from build123d import *

# Parameters (mm, degrees)
F1_DEPTH = 36
F3_DEPTH = 36
F4_R     = 14
F4_W     = 18
F4_H     = 16
F5_DEPTH = 44


with BuildPart() as f1:
    # F0 (on Front) → F1 (new body)
    with BuildSketch(Plane.XZ):
        Polygon((0, 44), (0, 0), (45, 0), (45, 13), (20, 27), (20, 44), align=None)
        Polygon((-45, 0), (0, 0), (0, 44), (-20, 44), (-20, 27), (-45, 13), align=None)
    extrude(amount=-F1_DEPTH)

    # F2 (on face) → F3 (cut)
    with BuildSketch(Plane.XZ):
        with BuildLine():
            Line((-20, 0), (20, 0))
            ThreePointArc((20, 0), (0, 20), (-20, 0))
        make_face()
    extrude(amount=-F3_DEPTH, mode=Mode.SUBTRACT)

    # F4 (on Top) → F5 (cut)
    with BuildSketch(Plane.XY):
        with Locations((0, 18)):
            Circle(F4_R)
        with Locations((-36.059196651, 18)):
            Rectangle(F4_W, F4_H)
        with Locations((36.059196651, 18)):
            Rectangle(F4_W, F4_H)
    extrude(amount=F5_DEPTH, mode=Mode.SUBTRACT)


solid = f1.part
Here's how the part is built. I have some questions about the finished solid (model axes, mm). A direction names the side the tool comes from. Round coordinates to 2 decimals unless told otherwise and drop trailing zeros. Loops run counter-clockwise (first coordinate to the right, second up) from the corner with the lowest first, then second, coordinate; pieces in that order, holes last. Notation, with made-up numbers: (49.25, 25.5) - (88.25, 25.5) arc R20 cw to (88.25, 51.5) - close; hole circle Ø9 at (-9.5, 48). An arc over 180 degrees is marked (long way). One line per question, with ' | ' between items. Start each with the question number.
Q1. I want a section at C-C (z = 33). Write out the boundary of the cut face in (x, y).
Q2. For faces 1 (the flat face through (-36, 26, 9)), 2 (the flat face through (36, 26, 9)), 3 (the flat face through (-20, 18, 36)), which set-ups out of +Z, -Z, +X, -X, +Y, -Y let a thin tool reach every point of the face, with its end or its side?
Q3. I want a section at B-B (x = 0). Write out the boundary of the cut face in (y, z).
Q4. Please list where these lines run through material, in increasing order: line 1 (X direction, y = 18, z = 38); line 2 (Y direction, x = 0, z = 30.25); line 3 (X direction, y = 6.5, z = 23). Write a range as [from, to].
Q5. I want a section at A-A (y = 18). Write out the boundary of the cut face in (x, z), then the cut area to 3 significant figures.
Q6. Will these pins go through, and if not, where does the flat tip stop? pin 1 (17.5 mm diameter, centred on y = 19.5, z = 6.5, fed in from +X); pin 2 (1 mm diameter, centred on y = 20, z = 20, fed in from -X); pin 3 (8.5 mm diameter, centred on y = 11.5, z = 38, fed in from +X); pin 4 (6 mm diameter, centred on y = 22, z = 22.5, fed in from +X).
Q7. I want a section at D-D (x = -32.5). Write out the boundary of the cut face in (y, z).
Response values:
1) outline: (-20, 0) - (20, 0) - (20, 36) - (-20, 36) - close; hole circle Ø28 at (0, 18)
2) face 1: +Z, -Z, -X | face 2: +Z, -Z, +X | face 3: +Z, -X, +Y, -Y
3) outline: (0, 20) - (4, 20) - (4, 44) - (0, 44) - close; (32, 20) - (36, 20) - (36, 44) - (32, 44) - close
4) line 1: x = [-20, -14], [14, 20] | line 2: y = [0, 4], [32, 36] | line 3: x = [-27.14, -7.98], [7.98, 27.14]
5) outline: (-27.06, 0) - (-20, 0) arc R20 cw to (-14, 14.28) - (-14, 44) - (-20, 44) - (-20, 27) - (-27.06, 23.05) - close; (14, 14.28) arc R20 cw to (20, 0) - (27.06, 0) - (27.06, 23.05) - (20, 27) - (20, 44) - (14, 44) - close | area: 763 mm²
6) pin 1: stops at x = 45 | pin 2: stops at x = -27.06 | pin 3: stops at x = 20 | pin 4: stops at x = 27.06
7) outline: (0, 0) - (10, 0) - (10, 20) - (0, 20) - close; (26, 0) - (36, 0) - (36, 20) - (26, 20) - close
